Check sheet for the modelled part. Datum: model origin and axes. Units: mm. A direction names the side the tool comes from. Give positions to 0.01 mm unless a question says otherwise; leave off trailing zeros. Order: outer loops, then holes, each group sorted by start corner. A loop starts at its lowest first (then second) coordinate and runs counter-clockwise, first axis right, second up.
```python
from build123d import *

# Parameters (mm, degrees)
F0_W     = 48.9
F0_H     = 81.9
F0_W_2   = 15
F0_H_2   = 5
F1_DEPTH = 2
F2_D     = 2
F2_DEPTH = 15
F2_TIP   = 0.600860619
F3_D     = 1
F3_DEPTH = 15
F3_TIP   = 0.3004303095
F4_SIZE  = 0.5


with BuildPart() as f1:
    # F0 (on Top) → F1 (new body)
    with BuildSketch(Plane.XY):
        Rectangle(F0_W, F0_H)
        with Locations((0, -24.5)):
            Rectangle(F0_W_2, F0_H_2, mode=Mode.SUBTRACT)
    extrude(amount=F1_DEPTH)

    # F2
    with Locations(Plane(origin=(0, 0, 0), x_dir=(1, 0, 0), z_dir=(0, 0, -1))):
        with Locations((-20.5, -37), (20.5, -37), (-20.5, 37), (20.5, 37)):
            Hole(F2_D / 2, depth=F2_DEPTH)
            with Locations((0, 0, -(F2_DEPTH + F2_TIP / 2))):  # 118° drill point
                Cone(0, F2_D / 2, F2_TIP, mode=Mode.SUBTRACT)

    # F3
    with Locations(Plane(origin=(0, 0, 0), x_dir=(1, 0, 0), z_dir=(0, 0, -1))):
        with Locations((-12.5, 24.5), (12.5, 24.5)):
            Hole(F3_D / 2, depth=F3_DEPTH)
            with Locations((0, 0, -(F3_DEPTH + F3_TIP / 2))):  # 118° drill point
                Cone(0, F3_D / 2, F3_TIP, mode=Mode.SUBTRACT)

    # F4
    f4_edges = [f1.edges().sort_by_distance(p)[0] for p in [
        (0, -22, 2),
        (-7.5, -24.5, 2),
        (0, -27, 2),
        (7.5, -24.5, 2),
    ]]
    chamfer(f4_edges, length=F4_SIZE)


solid = f1.part
```
(1) Gauge pin test, flat end, axial feed: pin 1 Ø1.6 at (x, y) = (20.5, 37) entering from -Z. Record the tip position at first contact, or that the pin passes through.
Response values:
pin 1: passes through
(2) Cross-section at A-A on x = 20.5. Enter the section's corners in (y, z), then the cut area to 3 significant figures.
Response values:
outline: (-40.95, 0) - (-38, 0) - (-38, 2) - (-40.95, 2) - close; (-36, 0) - (36, 0) - (36, 2) - (-36, 2) - close; (38, 0) - (40.95, 0) - (40.95, 2) - (38, 2) - close
area: 156 mm2
(3) Cross-section at D-D on z = 0.65. Enter the section's corners in (x, y).
Response values:
outline: (-24.45, -40.95) - (24.45, -40.95) - (24.45, 40.95) - (-24.45, 40.95) - close; hole circle Ø2 at (-20.5, -37); hole circle Ø2 at (-20.5, 37); hole circle Ø1 at (-12.5, -24.5); hole (-7.5, -27) - (7.5, -27) - (7.5, -22) - (-7.5, -22) - close; hole circle Ø1 at (12.5, -24.5); hole circle Ø2 at (20.5, -37); hole circle Ø2 at (20.5, 37)
(4) Set-up check for faces 5 (the face through (0, 40.95, 1)), 6 (the face through (7.5, -25, 1)): record each of +Z, -Z, +X, -X, +Y, -Y from which the full face is reachable in a straight line by a thin tool's end or side.
Response values:
face 5: +Z, -Z, +X, -X, +Y
face 6: +Z, -Z
(5) Cross-section at C-C on x = 5. Enter the section's corners in (y, z), then the cut area to 3 significant figures.
Response values:
outline: (-40.95, 0) - (-27, 0) - (-27, 1.5) - (-27.5, 2) - (-40.95, 2) - close; (-22, 0) - (40.95, 0) - (40.95, 2) - (-21.5, 2) - (-22, 1.5) - close
area: 154 mm2
(6) Release check for a two-part mould opening along X. For faces 1 (the face through (24.45, -1, 1)), 2 (the face through (0, 1, 0)), 3 (the face through (-24.45, -1, 1)), 4 (the face through (-7.5, -25, 1)) record: released by +X, released by -X, zero draft, split by the parting line, or undercut.
Response values:
face 1: released by +X
face 2: zero draft
face 3: released by -X
face 4: undercut
(7) Cross-section at B-B on y = -37. Enter the section's corners in (x, z), then the cut area to 3 significant figures.
Response values:
outline: (-24.45, 0) - (-21.5, 0) - (-21.5, 2) - (-24.45, 2) - close; (-19.5, 0) - (19.5, 0) - (19.5, 2) - (-19.5, 2) - close; (21.5, 0) - (24.45, 0) - (24.45, 2) - (21.5, 2) - close
area: 89.8 mm2
(8) Material ranges on L1, parallel to X at y = 37, z = 0.65; L2, parallel to X at y = -24.5, z = 0.6; L3, parallel to Y at x = -20.5, z = 0.65, recorded low to high.
Response values:
L1: x = -24.45 to -21.5, -19.5 to 19.5, 21.5 to 24.45
L2: x = -24.45 to -13, -12 to -7.5, 7.5 to 12, 13 to 24.45
L3: y = -40.95 to -38, -36 to 36, 38 to 40.95
